from build123d import *

# Parameters (mm, degrees)
SKETCH_2_W          = 150
SKETCH_2_H          = 290
EXTRUDE_1_DEPTH     = 3
SKETCH_3_W          = 42
SKETCH_3_H          = 74
CUT_EXTRUDE_1_DEPTH = 3
SKETCH_4_R          = 2.5
CUT_EXTRUDE_2_DEPTH = 3
SKETCH_5_W          = 30
SKETCH_5_H          = 110
CUT_EXTRUDE_3_DEPTH = 3
CUT_EXTRUDE_4_DEPTH = 3


with BuildPart() as part:
    # 草图2 → 凸台-拉伸1 (new body)
    with BuildSketch(Plane.XY):
        with Locations((46.825741224, -93.303848435)):
            Rectangle(SKETCH_2_W, SKETCH_2_H)
    extrude(amount=EXTRUDE_1_DEPTH)

    # 草图3 → 切除-拉伸1 (cut)
    with BuildSketch(Plane.XY.offset(3)):
        with Locations((48.825741224, -15.303848435)):
            Rectangle(SKETCH_3_W, SKETCH_3_H)
        with Locations((48.825741224, -151.303848435)):
            Rectangle(SKETCH_3_W, SKETCH_3_H)
    extrude(amount=-CUT_EXTRUDE_1_DEPTH, mode=Mode.SUBTRACT)

    # 草图4 → 切除-拉伸2 (cut)
    with BuildSketch(Plane.XY.offset(3)):
        with Locations((-18.174258776, 41.696151565)):
            Circle(SKETCH_4_R)
        with Locations((-18.174258776, -228.303848435)):
            Circle(SKETCH_4_R)
    extrude(amount=-CUT_EXTRUDE_2_DEPTH, mode=Mode.SUBTRACT)

    # 草图5 → 切除-拉伸3 (cut)
    with BuildSketch(Plane.XY.offset(3)):
        with Locations((5.068322333, -16.872516049)):
            Rectangle(SKETCH_5_W, SKETCH_5_H)
        with Locations((93.246188271, -16.872516049)):
            Rectangle(SKETCH_5_W, SKETCH_5_H)
        with Locations((5.068322333, -159.262913685)):
            Rectangle(SKETCH_5_W, SKETCH_5_H)
        with Locations((93.246188271, -159.262913685)):
            Rectangle(SKETCH_5_W, SKETCH_5_H)
    extrude(amount=-CUT_EXTRUDE_3_DEPTH, mode=Mode.SUBTRACT)

    # 草图6 → 切除-拉伸4 (cut)
    with BuildSketch(Plane.XY.offset(3)):
        with BuildLine():
            Line((5.068322333, -219.315553818), (105.068322333, -219.315553818))
            ThreePointArc((105.068322333, -219.315553818), (110.068322333, -224.315553818), (105.068322333, -229.315553818))
            Line((105.068322333, -229.315553818), (5.068322333, -229.315553818))
            ThreePointArc((5.068322333, -229.315553818), (0.068322333, -224.315553818), (5.068322333, -219.315553818))
        make_face()
    extrude(amount=-CUT_EXTRUDE_4_DEPTH, mode=Mode.SUBTRACT)


solid = part.part
Work out the finished part from the listing and answer in its coordinate system (mm). A direction names the side the tool comes from. Give positions to 0.01 mm unless a question says otherwise; leave off trailing zeros. Loops run counter-clockwise (first coordinate to the right, second up) from the corner with the lowest first, then second, coordinate; pieces in that order, holes last. Notation, with made-up numbers: (17.5, 73.25) -> (67.5, 73.25) arc R29 ccw to (67.5, 98.25) -> close; hole circle Ø5 at (-28, -27). An arc over 180 degrees is marked (long way). Use a Markdown table: item, result. Add a question column.
1. Section C-C on x = 50 is taken. Determine the outline of the cut face in (y, z).
2. Determine the mould class of faces 1 (the flat face through (46, -91, 3)), 2 (the cylindrical face through (-20.017, 43.386, 1.521)), 3 (the cylindrical face through (-18.5, -225.825, 1.521)) for opening direction Y: released by +Y, released by -Y, zero draft, split by the parting line, or undercut.
3. Section A-A on x = -6 is taken. Determine the outline of the cut face in (y, z).
4. Section D-D on z = 2.5 is taken. State how many separate pieces and enclosed holes the cut face has, and give its area (3 significant figures).
5. A flat-ended cylindrical pin translates along its axis: pin 1 Ø6.5 at (x, y) = (-18.17, -228.3) entering from -Z. Find the tip coordinate at first contact, or state that the pin passes through.
6. For faces 4 (the flat face through (46, -91, 0)), 5 (the cylindrical face through (0.07, -224.43, 1.52)), determine the directions among +Z, -Z, +X, -X, +Y, -Y from which every point of the face is accessible in a straight line to the end or side of a thin tool.
7. Find the intervals of material crossed by probe 1 along Y at (x, z) = (49, 0.75); probe 2 along X at (y, z) = (-158, 2.35); probe 3 along Y at (x, z) = (103, 2.85), in increasing order.
8. Section B-B on y = -183 is taken. Determine the outline of the cut face in (x, z), and give its area (3 significant figures).
Results below:
| question | item | result |
|---|---|---|
| 1 | outline | (-238.3, 0) -> (-229.32, 0) -> (-229.32, 3) -> (-238.3, 3) -> close; (-219.32, 0) -> (-188.3, 0) -> (-188.3, 3) -> (-219.32, 3) -> close; (-114.3, 0) -> (-52.3, 0) -> (-52.3, 3) -> (-114.3, 3) -> close; (21.7, 0) -> (51.7, 0) -> (51.7, 3) -> (21.7, 3) -> close |
| 2 | face 1 | zero draft |
| 2 | face 2 | undercut |
| 2 | face 3 | undercut |
| 3 | outline | (-238.3, 0) -> (-214.26, 0) -> (-214.26, 3) -> (-238.3, 3) -> close; (-104.26, 0) -> (-71.87, 0) -> (-71.87, 3) -> (-104.26, 3) -> close; (38.13, 0) -> (51.7, 0) -> (51.7, 3) -> (38.13, 3) -> close |
| 4 | separate pieces | 1 |
| 4 | enclosed holes | 9 |
| 4 | area | 23,000 mm^2 |
| 5 | pin 1 | stops at z = 0 |
| 6 | face 4 | -Z, +X, -X, +Y, -Y |
| 6 | face 5 | +Z, -Z |
| 7 | probe 1 | y = -238.3 to -229.32, -219.32 to -188.3, -114.3 to -52.3, 21.7 to 51.7 |
| 7 | probe 2 | x = -28.17 to -9.93, 20.07 to 27.83, 69.83 to 78.25, 108.25 to 121.83 |
| 7 | probe 3 | y = -238.3 to -229.32, -219.32 to -214.26, -104.26 to -71.87, 38.13 to 51.7 |
| 8 | outline | (-28.17, 0) -> (-9.93, 0) -> (-9.93, 3) -> (-28.17, 3) -> close; (20.07, 0) -> (27.83, 0) -> (27.83, 3) -> (20.07, 3) -> close; (69.83, 0) -> (78.25, 0) -> (78.25, 3) -> (69.83, 3) -> close; (108.25, 0) -> (121.83, 0) -> (121.83, 3) -> (108.25, 3) -> close |
| 8 | area | 144 mm^2 |
